Source: CAD feature listing. Evaluate the final solid. Frame: model axes, mm. A direction names the side the tool comes from. Give positions to 0.01 mm unless a question says otherwise; leave off trailing zeros. Write each loop counter-clockwise with the first axis right and the second up, starting at its lowest first coordinate (ties: lowest second). Pieces come first, ordered by that corner, then holes. Notation, with made-up numbers: (16, 6) -> (65, 6) arc R23 ccw to (65, 43) -> close; hole circle Ø9 at (70, 88.5). An arc over 180 degrees is marked (long way). Answer as a JSON object with one key per item and string values. Group by question number.
Item 1: Section query C-C on y = 83. Return the cut outline in (x, z).
Item 2: Section query A-A on y = 32. Return the cut outline in (x, z).
Item 3: Section query D-D on x = 3.5. Give the number of separate pieces and of enclosed holes in the cut face, plus the area to 3 significant figures.
Item 4: Pull-direction query (Y, two-part tool) for faces 5 (the face through (2, 86.05, 52)), 6 (the face through (2, 56.5, -3)), 7 (the face through (5, 46, 23)); classes: pulls with the +Y half, pulls with the -Y half, needs draft (parallel to the pull), parting line crosses it, or undercut.
Item 5: Access query for faces 1 (the face through (2, 36.5, 89)), 2 (the face through (2, 74, 0)), 3 (the face through (2, 46, 77.6)), 4 (the face through (2, 95, 53.5)). Directions: +Z, -Z, +X, -X, +Y, -Y. A direction counts if a zero-diameter tool reaches every point of the face in a straight line with its end or side. Return the directions, or none.
Item 6: Section query B-B on z = 35. Return the cut outline in (x, y), plus the area to 4 significant figures.
Item 7: First-contact query: pin 1 Ø2.5 at (x, z) = (3.5, -2.5) entering from +Y; pin 2 Ø1.5 at (x, z) = (3.5, 63) entering from +Y; pin 3 Ø2.5 at (x, y) = (2.5, 82.5) entering from +Z. Flat tips, straight axial feed; report the tip coordinate or a pass-through.
Item 8: Ray query, probe 1 along Z at (x, y) = (1.95, 65); probe 2 along Y at (x, z) = (1.2, 84.4); probe 3 along Z at (x, y) = (4.5, 17.5). Return the intervals inside material, ascending. Write a range as from..to.
from build123d import *

# Parameters (mm, degrees)
F1_R     = 1.6
F1_R_2   = 6.5
F1_R_3   = 3.5
F1_W     = 78.7
F1_H     = 51.25
F1_W_2   = 20
F1_H_2   = 5
F1_W_3   = 5
F1_H_3   = 20
F2_DEPTH = 5


with BuildPart() as f2:
    # F1 (on Right) → F2 (new body)
    with BuildSketch(Plane.YZ):
        Polygon((36.5, 87), (0, 87), (0, 53.5), (0, 33.5), (0, 0), (36.5, 0), (56.5, 0), (93, 0), (93, 33.5), (93, 53.5), (93, 87), (56.5, 87), align=None)
        with Locations((2.5, 19.4)):
            Circle(F1_R, mode=Mode.SUBTRACT)
        with Locations((65.25, 8)):
            Circle(F1_R_2, mode=Mode.SUBTRACT)
        with Locations((83, 8)):
            Circle(F1_R_3, mode=Mode.SUBTRACT)
        with Locations((90.5, 19.4)):
            Circle(F1_R, mode=Mode.SUBTRACT)
        with Locations((2.5, 84.4)):
            Circle(F1_R, mode=Mode.SUBTRACT)
        with Locations((46.7, 51.975)):
            Rectangle(F1_W, F1_H, mode=Mode.SUBTRACT)
        with Locations((90.5, 84.4)):
            Circle(F1_R, mode=Mode.SUBTRACT)
        with Locations((46.5, 89.5)):
            Rectangle(F1_W_2, F1_H_2)
        with Locations((-2.5, 43.5)):
            Rectangle(F1_W_3, F1_H_3)
        with Locations((95.5, 43.5)):
            Rectangle(F1_W_3, F1_H_3)
        with Locations((46.5, -2.5)):
            Rectangle(F1_W_2, F1_H_2)
    extrude(amount=F2_DEPTH)


solid = f2.part
Worked answers:
{
 "1": {"outline": "(0, 0) -> (5, 0) -> (5, 4.5) -> (0, 4.5) -> close; (0, 11.5) -> (5, 11.5) -> (5, 26.35) -> (0, 26.35) -> close; (0, 77.6) -> (5, 77.6) -> (5, 87) -> (0, 87) -> close"},
 "2": {"outline": "(0, 0) -> (5, 0) -> (5, 26.35) -> (0, 26.35) -> close; (0, 77.6) -> (5, 77.6) -> (5, 87) -> (0, 87) -> close"},
 "3": {"separate pieces": "1", "enclosed holes": "7", "area": "4,250 mm^2"},
 "4": {"face 5": "undercut", "face 6": "pulls with the +Y half", "face 7": "needs draft"},
 "5": {"face 1": "+Z, +X, -X, -Y", "face 2": "-Z, +X, -X, +Y", "face 3": "+X, -X", "face 4": "+Z, +X, -X, +Y"},
 "6": {"outline": "(0, -5) -> (5, -5) -> (5, 7.35) -> (0, 7.35) -> close; (0, 86.05) -> (5, 86.05) -> (5, 98) -> (0, 98) -> close", "area": "121.5 mm^2"},
 "7": {"pin 1": "y = 56.5", "pin 2": "y = 93", "pin 3": "z = 87"},
 "8": {"probe 1": "0..1.5, 14.5..26.35, 77.6..87", "probe 2": "0..0.9, 4.1..88.9, 92.1..93", "probe 3": "0..26.35, 77.6..87"}
}
